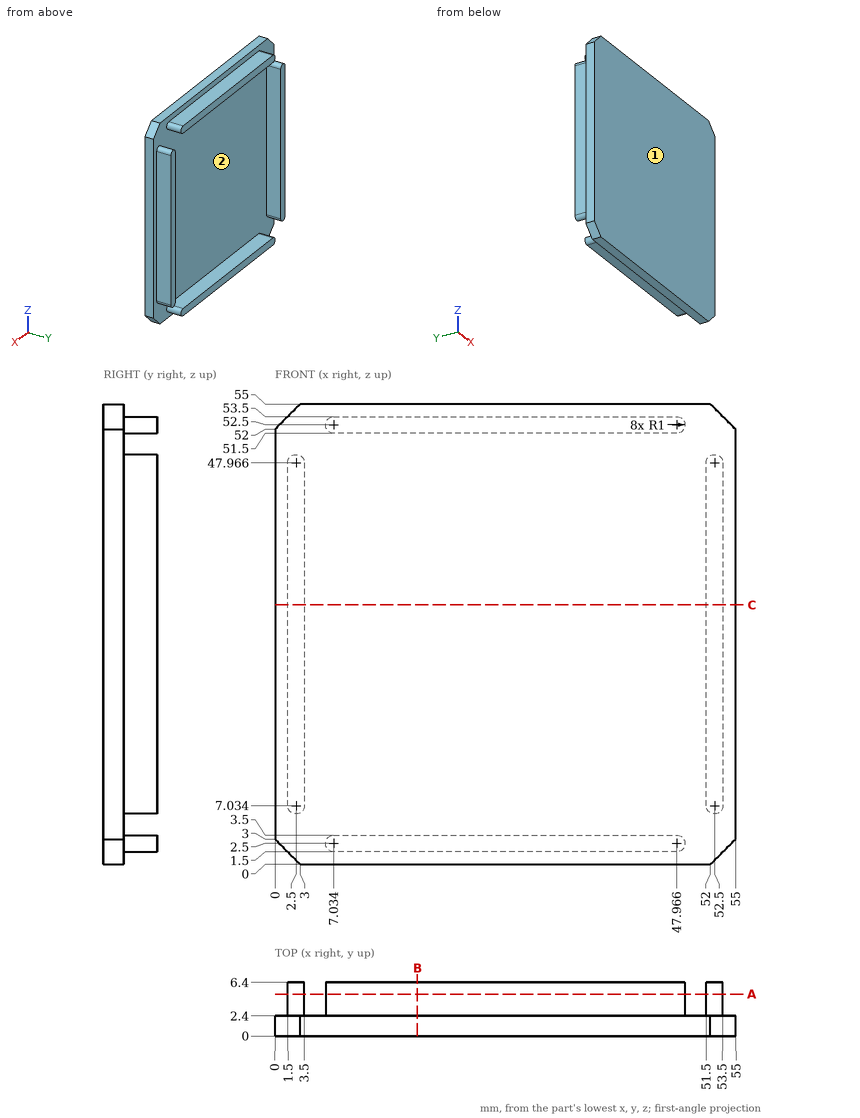
Could you check a few things on this drawing? It's one solid part, dimensions in mm from its lowest x, y, z. Coordinates: 2 decimals unless noted, no trailing zeros. Loops run counter-clockwise (first coordinate to the right, second up) from the corner with the lowest first, then second, coordinate; pieces in that order, holes last.
1. Imagine slicing it at A-A (y = 5). Please give me the cut outline in (x, z) (1 decimal).
2. For P1, Ø5, axis at x = 36, z = 44.5, coming from the +Y side; P2, Ø3, axis at y = 4, z = 24.5, coming from the -X side; P3, Ø3, axis at x = 33.5, y = 5, coming from the -Z side, each with a flat end and sliding along its axis, tell me the tip position at first contact or that it passes through.
3. I need wall thicknesses on L1, parallel to X at y = 3.75, z = 25.5; L2, parallel to Y at x = 28, z = 32. Which ranges of each line are inside material? Lowest first, please.
4. We'd pull the mould along Z, two halves only. Please class the marked faces 1 and 2: released by +Z, released by -Z, zero draft, split by the parting line, or undercut.
5. Imagine slicing it at C-C (z = 31). Please give me the cut outline in (x, y), and give its area (3 significant figures).
6. Imagine slicing it at B-B (x = 17). Please give me the cut outline in (y, z).
Computed values:
1. outline: (1.5, 7) arc R1 ccw to (3.5, 7) - (3.5, 48) arc R1 ccw to (1.5, 48) - close; (7, 1.5) - (48, 1.5) arc R1 ccw to (48, 3.5) - (7, 3.5) arc R1 ccw to start; (7, 51.5) - (48, 51.5) arc R1 ccw to (48, 53.5) - (7, 53.5) arc R1 ccw to start; (51.5, 7) arc R1 ccw to (53.5, 7) - (53.5, 48) arc R1 ccw to (51.5, 48) - close
2. P1: stops at y = 2.4
2. P2: stops at x = 1.5
2. P3: stops at z = 1.5
3. L1: x = 1.5 to 3.5, 51.5 to 53.5
3. L2: y = 0 to 2.4
4. face 1: zero draft
4. face 2: undercut
5. outline: (0, 0) - (55, 0) - (55, 2.4) - (53.5, 2.4) - (53.5, 6.4) - (51.5, 6.4) - (51.5, 2.4) - (3.5, 2.4) - (3.5, 6.4) - (1.5, 6.4) - (1.5, 2.4) - (0, 2.4) - close
5. area: 148 mm2
6. outline: (0, 0) - (2.4, 0) - (2.4, 1.5) - (6.4, 1.5) - (6.4, 3.5) - (2.4, 3.5) - (2.4, 51.5) - (6.4, 51.5) - (6.4, 53.5) - (2.4, 53.5) - (2.4, 55) - (0, 55) - close
